Read the model definition and answer for the solid it produces. Units are mm, in the model's axes. A direction names the side the tool comes from. Give positions to 0.01 mm unless a question says otherwise; leave off trailing zeros. Loops run counter-clockwise (first coordinate to the right, second up) from the corner with the lowest first, then second, coordinate; pieces in that order, holes last. Notation, with made-up numbers: (-16, 25.5) -> (-8, 25.5) arc R12 ccw to (-8, 40.5) -> close; hole circle Ø4 at (20.5, 1.25). An arc over 180 degrees is marked (long way). One line per item, written item: value. Start each with the question number.
from build123d import *

# Parameters (mm, degrees)
SKETCH2_W           = 20
SKETCH2_H           = 3
BOSS_EXTRUDE1_DEPTH = 1.5875
SKETCH3_R           = 6
BOSS_EXTRUDE2_DEPTH = 3.175
SKETCH4_R           = 2.6
CUT_EXTRUDE1_DEPTH  = 24.023479863
BOSS_EXTRUDE3_DEPTH = 3.175
FILLET1_R           = 2.5


with BuildPart() as part:
    # Sketch2 → Boss-Extrude1 (new, symmetric)
    with BuildSketch(Plane.XY):
        with BuildLine():
            Line((10, 3.5), (10, -3.5))
            ThreePointArc((10, -3.5), (13.5, 0), (10, 3.5))
        make_face()
        Rectangle(SKETCH2_W, SKETCH2_H)
    extrude(amount=BOSS_EXTRUDE1_DEPTH, both=True)



with BuildPart() as body_2:
    # Sketch3 → Boss-Extrude2 (new body)
    with BuildSketch(Plane.XY.offset(1.5875)):
        with Locations((-16, 0)):
            Circle(SKETCH3_R)
    extrude(amount=-BOSS_EXTRUDE2_DEPTH)

    # Sketch4 → Cut-Extrude1 (cut, through all)
    with BuildSketch(Plane.XY.offset(1.5875)):
        with Locations((-16, 0)):
            Circle(SKETCH4_R)
    extrude(amount=-CUT_EXTRUDE1_DEPTH, mode=Mode.SUBTRACT)


with BuildPart() as part_1:
    add(part.part)

    add(body_2.part)  # Boss-Extrude3 merges body 2
    # Sketch6 → Boss-Extrude3 (add)
    with BuildSketch(Plane.XY.offset(1.5875)):
        Polygon((-10, -1.5), (-10, 0), (-10.190524981, -1.5), align=None)
    boss_extrude3 = extrude(amount=-BOSS_EXTRUDE3_DEPTH)

    # Mirror1: Boss-Extrude3 across plane
    add(boss_extrude3.mirror(Plane.ZX))

    # Fillet1
    fillet1_edges = [part_1.edges().sort_by_distance(p)[0] for p in [
        (-10.190524981, -1.5, 0),
        (-10.190524981, 1.5, 0),
    ]]
    fillet(fillet1_edges, radius=FILLET1_R)


solid = part_1.part
Item 1: Flat-ended cylindrical pins translate along their axes: pin 1 (1.6 mm diameter, centred on x = -1.5, z = -0.5, fed in from +Y); pin 2 (1.6 mm diameter, centred on y = 2, z = 0, fed in from -X); pin 3 (1.5 mm diameter, centred on y = -3.5, z = 0, fed in from -X). Find the tip coordinate at first contact, or state that the pin passes through.
Item 2: Section B-B, the plane y = 0 is taken. Determine the outline of the cut face in (x, z).
Item 3: For faces 1 (the cylindrical face through (-22, 0, 0)), 2 (the flat face through (10, 3, 0)), 3 (the cylindrical face through (-10, -2, 0)), determine the directions among +Z, -Z, +X, -X, +Y, -Y from which every point of the face is accessible in a straight line to the end or side of a thin tool.
Item 4: Consider L1, parallel to Y at x = -16, z = 0.5; L2, parallel to Y at x = 5, z = 0.1; L3, parallel to X at y = 1, z = 0.5. Determine where each line is inside the solid, lowest interval first. Write a range as [from, to].
Item 5: Section C-C, the plane z = 0.9 is taken. Determine the outline of the cut face in (x, y), plus the area to 3 significant figures.
Item 6: Determine the mould class of faces 4 (the flat face through (1, 1.5, 0)), 5 (the cylindrical face through (13.5, -0.1, 0)), 6 (the flat face through (-8, 0, -1.588)) for opening direction X: pulls with the +X half, pulls with the -X half, needs draft (parallel to the pull), parting line crosses it, or undercut.
Item 7: Section D-D, the plane x = -2.5 is taken. Determine the outline of the cut face in (y, z), plus the area to 4 significant figures.
Item 8: Section A-A, the plane x = -16 is taken. Determine the outline of the cut face in (y, z), plus the area to 3 significant figures.
Computed values:
1. pin 1: y = 1.5
1. pin 2: x = -21.88
1. pin 3: x = -21.33
2. outline: (-22, -1.59) -> (-18.6, -1.59) -> (-18.6, 1.59) -> (-22, 1.59) -> close; (-13.4, -1.59) -> (13.5, -1.59) -> (13.5, 1.59) -> (-13.4, 1.59) -> close
3. face 1: +Z, -Z
3. face 2: +Z, -Z, +Y
3. face 3: +Z, -Z, -Y
4. L1: [-6, -2.6], [2.6, 6]
4. L2: [-1.5, 1.5]
4. L3: [-21.92, -18.4], [-13.6, 13.35]
5. outline: (-10.71, -2.82) arc R2.5 cw to (-8.5, -1.5) -> (10, -1.5) -> (10, -3.5) arc R3.5 ccw to (10, 3.5) -> (10, 1.5) -> (-8.5, 1.5) arc R2.5 cw to (-10.71, 2.82) arc R6 ccw (long way) to start; hole circle Ø5.2 at (-16, 0)
5. area: 172 mm²
6. face 4: undercut
6. face 5: pulls with the +X half
6. face 6: needs draft
7. outline: (-1.5, -1.59) -> (1.5, -1.59) -> (1.5, 1.59) -> (-1.5, 1.59) -> close
7. area: 9.525 mm²
8. outline: (-6, -1.59) -> (-2.6, -1.59) -> (-2.6, 1.59) -> (-6, 1.59) -> close; (2.6, -1.59) -> (6, -1.59) -> (6, 1.59) -> (2.6, 1.59) -> close
8. area: 21.6 mm²
